from build123d import *

# Parameters (mm, degrees)
SKETCH_1_W          = 20
SKETCH_1_H          = 20
EXTRUDE_1_DEPTH     = 290
SKETCH_2_R          = 2.15
SKETCH_2_R_2        = 2
CUT_EXTRUDE_1_DEPTH = 291.344622819
HOLE_WIZARD_M6_1_D  = 6.6


with BuildPart() as part:
    # 스케치1 → 보스-돌출1 (new body)
    with BuildSketch(Plane.XY):
        Rectangle(SKETCH_1_W, SKETCH_1_H)
    extrude(amount=EXTRUDE_1_DEPTH)

    # 스케치2 → 컷-돌출1 (cut, through all)
    with BuildSketch(Plane.XY.offset(290)):
        Circle(SKETCH_2_R)
        with Locations((-7, 7)):
            Circle(SKETCH_2_R_2)
        with Locations((7, 7)):
            Circle(SKETCH_2_R_2)
        with Locations((7, -7)):
            Circle(SKETCH_2_R_2)
        with Locations((-7, -7)):
            Circle(SKETCH_2_R_2)
        with BuildLine():
            Line((-2.65, 10), (-2.65, 8.5))
            Line((-2.65, 8.5), (-4.15, 8.5))
            Line((-4.15, 8.5), (-4.15, 5.5))
            ThreePointArc((-4.15, 5.5), (0, 4), (4.15, 5.5))
            Line((4.15, 5.5), (4.15, 8.5))
            Line((4.15, 8.5), (2.65, 8.5))
            Line((2.65, 8.5), (2.65, 10))
            Line((2.65, 10), (-2.65, 10))
        make_face()
        with BuildLine():
            Line((10, 2.65), (8.5, 2.65))
            Line((8.5, 2.65), (8.5, 4.15))
            Line((8.5, 4.15), (5.5, 4.15))
            ThreePointArc((5.5, 4.15), (4, 0), (5.5, -4.15))
            Line((5.5, -4.15), (8.5, -4.15))
            Line((8.5, -4.15), (8.5, -2.65))
            Line((8.5, -2.65), (10, -2.65))
            Line((10, -2.65), (10, 2.65))
        make_face()
        with BuildLine():
            Line((2.65, -10), (2.65, -8.5))
            Line((2.65, -8.5), (4.15, -8.5))
            Line((4.15, -8.5), (4.15, -5.5))
            ThreePointArc((4.15, -5.5), (0, -4), (-4.15, -5.5))
            Line((-4.15, -5.5), (-4.15, -8.5))
            Line((-4.15, -8.5), (-2.65, -8.5))
            Line((-2.65, -8.5), (-2.65, -10))
            Line((-2.65, -10), (2.65, -10))
        make_face()
        with BuildLine():
            Line((-10, -2.65), (-8.5, -2.65))
            Line((-8.5, -2.65), (-8.5, -4.15))
            Line((-8.5, -4.15), (-5.5, -4.15))
            ThreePointArc((-5.5, -4.15), (-4, 0), (-5.5, 4.15))
            Line((-5.5, 4.15), (-8.5, 4.15))
            Line((-8.5, 4.15), (-8.5, 2.65))
            Line((-8.5, 2.65), (-10, 2.65))
            Line((-10, 2.65), (-10, -2.65))
        make_face()
    extrude(amount=-CUT_EXTRUDE_1_DEPTH, mode=Mode.SUBTRACT)

    # M6 여유 구멍1 (through all)
    with Locations(Plane.ZY.offset(10)):
        with Locations((10, 0), (280, 0)):
            Hole(HOLE_WIZARD_M6_1_D / 2)


solid = part.part
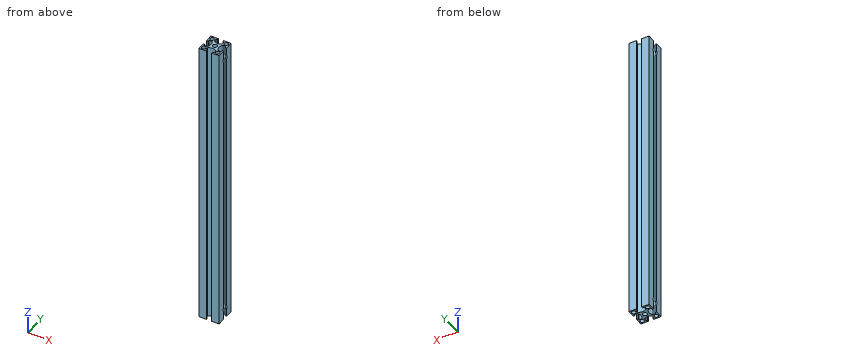
For this review, take the finished solid that the model builds, in its own axes (mm). Give positions to 0.01 mm unless a question says otherwise; leave off trailing zeros. Answer as a JSON object with one key per item and string values. Group by question number.
Item 1: Wall thickness on line 1 along Y through (x, z) = (-7, 59.5); line 2 along X through (y, z) = (0, 224); line 3 along Y through (x, z) = (-5.25, 160): over which ranges is each line inside the solid? List them lowest first.
Item 2: Take a section at A-A on z = 72. Give the number of separate pieces and of enclosed holes in the cut face, and give its area (3 significant figures).
Item 3: Clearance check with flat-ended pins moving along their axes: pin 1 Ø8 at (x, y) = (-3, 7.5) entering from -Z; pin 2 Ø2 at (y, z) = (1, 83) entering from -X; pin 3 Ø3 at (x, y) = (-7, -7) entering from -Z (3 decimals). State where each tip first meets the part, or that it passes through.
Reported:
{
 "1": {"line 1": "-10 to -9, -5 to -4.15, 4.15 to 5, 9 to 10", "line 2": "-4 to -2.15, 2.15 to 4", "line 3": "-10 to -7.97, -6.03 to -3.83, 3.83 to 6.03, 7.97 to 10"},
 "2": {"separate pieces": "1", "enclosed holes": "5", "area": "170 mm^2"},
 "3": {"pin 1": "z = 0", "pin 2": "x = -4.32", "pin 3": "through"}
}
